Model file for the job. Use its own axes, mm. A direction names the side the tool comes from. Give positions to 0.01 mm unless a question says otherwise; leave off trailing zeros. Order: outer loops, then holes, each group sorted by start corner. A loop starts at its lowest first (then second) coordinate and runs counter-clockwise, first axis right, second up. Notation, with made-up numbers: M 72.25,62.5 L 112.25,62.5 A26 ccw 112.25,78.5 Z; hole C 31.25,-18.5 d3. An arc over 180 degrees is marked long. Return JSON: item names as keys, results as strings. Group by question number.
1. Pin check, flat tips, straight feed: pin 1 (1 mm diameter, centred on x = 7.5, y = 4.5, fed in from +Z); pin 2 (1 mm diameter, centred on y = -8, z = 2.5, fed in from +X). Stop position of each tip, or through.
2. Slice it at B-B on x = -7. List the corners of the cut face in (y, z), then the cut area to 3 significant figures.
3. 3-axis set-ups, long thin cutter, end or side, ignore diameter. For faces 4 (the face through (-0.17, 1.29, 2.03)), 5 (the face through (-6.99, -0.87, 3.04)), 6 (the face through (0, -2, 1)): which of +Z, -Z, +X, -X, +Y, -Y reach the whole face in a straight line?
4. Wall check: probe 1 along Y at (x, z) = (-6.5, 3.65); probe 2 along Y at (x, z) = (0, 2.1); probe 3 along Z at (x, y) = (-5, 0.5). Give the ranges that are in metal, low to high. Write a range as [from, to].
5. Two-plate mould, pull along Y, no slides. Class faces 1 (the face through (0, -4, 0)), 2 (the face through (12.58, 7.21, 3.04)), 3 (the face through (-13.887, -10.648, 1.864)): released by +Y, released by -Y, zero draft, split by the parting line, or undercut.
6. Slice it at C-C on z = 3.1. List the corners of the cut face in (x, y) (3 decimals), then the cut area to 3 significant figures.
7. Slice it at A-A on y = -11.5. List the corners of the cut face in (x, z), then the cut area to 3 significant figures.
8. Slice it at D-D on x = 0. List the corners of the cut face in (y, z).
from build123d import *

# Parameters (mm, degrees)
SCHIZZO1_R                   = 17.5
ESTRUSIONE_ESTRUSIONE1_DEPTH = 3.781092502
SCHIZZO2_R                   = 1.625
SCHIZZO2_R_2                 = 1.3
TAGLIO_ESTRUSIONE1_DEPTH     = 4.781092502
CUT_EXTRUDE1_DEPTH           = 1.5
SCHIZZO4_R                   = 2
TAGLIO_ESTRUSIONE2_DEPTH     = 1.781093


with BuildPart() as part:
    # Schizzo1 → Estrusione-Estrusione1 (new body)
    with BuildSketch(Plane.XY):
        Circle(SCHIZZO1_R)
    extrude(amount=ESTRUSIONE_ESTRUSIONE1_DEPTH)

    # Schizzo2 → Taglio-Estrusione1 (cut, through all)
    with BuildSketch(Plane.XY.offset(3.781092502)):
        with Locations((12, 0)):
            Circle(SCHIZZO2_R)
        with Locations((-6, 10.392304845)):
            Circle(SCHIZZO2_R)
        with Locations((-6, -10.392304845)):
            Circle(SCHIZZO2_R)
        Circle(SCHIZZO2_R_2)
    extrude(amount=-TAGLIO_ESTRUSIONE1_DEPTH, mode=Mode.SUBTRACT)

    # Sketch1 → Cut-Extrude1 (cut)
    with BuildSketch(Plane.XY.offset(3.781092502)):
        with BuildLine():
            Line((2.10108498, -2.799185936), (12.025937536, 4.650465179))
            ThreePointArc((12.025937536, 4.650465179), (12.557368355, 7.25), (10.040389753, 8.089534821))
            Line((10.040389753, 8.089534821), (-1.373623641, 3.219185936))
            ThreePointArc((-1.373623641, 3.219185936), (-1.75, 3.031088913), (-2.10108498, 2.799185936))
            Line((-2.10108498, 2.799185936), (-12.025937536, -4.650465179))
            ThreePointArc((-12.025937536, -4.650465179), (-12.557368355, -7.25), (-10.040389753, -8.089534821))
            Line((-10.040389753, -8.089534821), (1.373623641, -3.219185936))
            ThreePointArc((1.373623641, -3.219185936), (1.75, -3.031088913), (2.10108498, -2.799185936))
        make_face()
    extrude(amount=-CUT_EXTRUDE1_DEPTH, mode=Mode.SUBTRACT)

    # Schizzo4 → Taglio-Estrusione2 (cut)
    with BuildSketch(Plane(origin=(0, 0, 0), x_dir=(-1, 0, 0), z_dir=(0, 0, -1))):
        Circle(SCHIZZO4_R)
    extrude(amount=-TAGLIO_ESTRUSIONE2_DEPTH, mode=Mode.SUBTRACT)


solid = part.part
Result:
{
 "1": {"pin 1": "stops at z = 2.28", "pin 2": "stops at x = 15.81"},
 "2": {"outline": "M -16.04,0 L -11.67,0 L -11.67,3.78 L -16.04,3.78 Z; M -9.11,0 L 9.11,0 L 9.11,3.78 L -0.88,3.78 L -0.88,2.28 L -6.79,2.28 L -6.79,3.78 L -9.11,3.78 Z; M 11.67,0 L 16.04,0 L 16.04,3.78 L 11.67,3.78 Z", "area": "93.0 mm2"},
 "3": {"face 4": "+Z, -Z", "face 5": "+Z", "face 6": "-Z"},
 "4": {"probe 1": "y = [-16.25, -11.94], [-8.85, -6.58], [-0.5, 8.85], [11.94, 16.25]", "probe 2": "y = [-17.5, -1.3], [1.3, 17.5]", "probe 3": "z = [0, 2.28]"},
 "5": {"face 1": "zero draft", "face 2": "undercut", "face 3": "split by the parting line"},
 "6": {"outline": "C 0,0 d35; hole M -12.026,-4.65 A2 ccw -10.04,-8.09 L 1.374,-3.219 A3.5 ccw 2.101,-2.799 L 12.026,4.65 A2 ccw 10.04,8.09 L -1.374,3.219 A3.5 ccw -2.101,2.799 Z; hole C -6,-10.392 d3.25; hole C -6,10.392 d3.25; hole C 12,0 d3.25", "area": "786 mm2"},
 "7": {"outline": "M -13.19,0 L -7.19,0 L -7.19,3.78 L -13.19,3.78 Z; M -4.81,0 L 13.19,0 L 13.19,3.78 L -4.81,3.78 Z", "area": "90.8 mm2"},
 "8": {"outline": "M -17.5,0 L -2,0 L -2,1.78 L -1.3,1.78 L -1.3,2.28 L -3.81,2.28 L -3.81,3.78 L -17.5,3.78 Z; M 1.3,1.78 L 2,1.78 L 2,0 L 17.5,0 L 17.5,3.78 L 3.81,3.78 L 3.81,2.28 L 1.3,2.28 Z"}
}
